Can you work these out from the drawing? Everything is in mm from the part's minimum corner. A direction names the side the tool comes from. Give positions to 0.01 mm unless a question says otherwise; leave off trailing zeros. Loops run counter-clockwise (first coordinate to the right, second up) from the corner with the lowest first, then second, coordinate; pieces in that order, holes last. Notation, with made-up numbers: (53, 30) - (81, 30) arc R17 ccw to (81, 63) - close; hole circle Ø9 at (52.25, -9). An arc over 180 degrees is marked (long way). One line per item, written item: value. Start each with the question number.
Q1. I want a section at C-C (x = 11.5). Please give me the cut outline in (y, z).
Q2. For the marked faces 1 and 2, which set-ups out of +Z, -Z, +X, -X, +Y, -Y let a thin tool reach every point of the face, with its end or its side?
Q3. I'm going to push flat-ended pins straight in: P1, Ø4, axis at y = 5.5, z = 64, coming from the +X side; P2, Ø6, axis at x = 16.5, y = 10.5, coming from the +Z side. Where does each tip first touch, or does it pass through?
Q4. If I drill on line 1 (Y direction, x = 22.5, z = 4.25); line 2 (X direction, y = 15, z = 48), over which ranges is the centre line in solid material (lowest first)? Write a range as from..to.
Q5. I want a section at D-D (z = 21.5). Please give me the cut outline in (x, y), then the cut area to 3 significant figures.
Q6. I want a section at A-A (x = 22.5). Please give me the cut outline in (y, z).
Q7. I want a section at B-B (y = 12.5). Please give me the cut outline in (x, z).
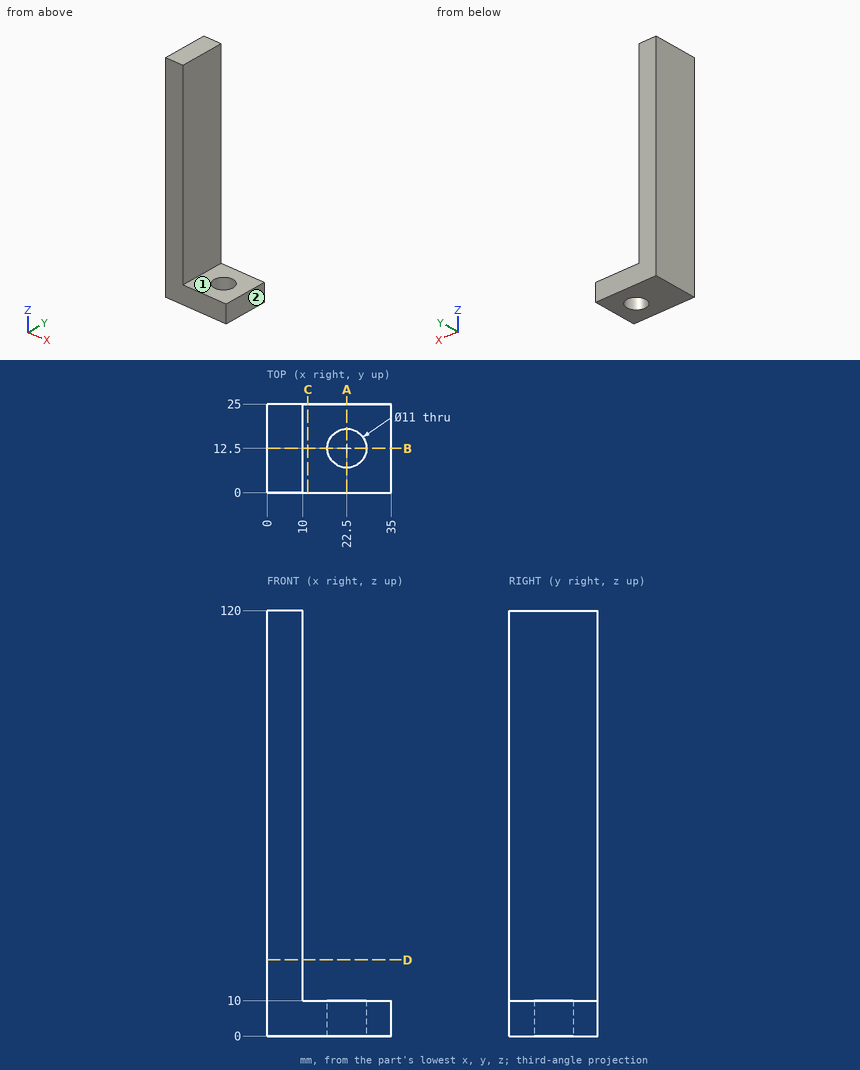
Worked answers:
1. outline: (0, 0) - (25, 0) - (25, 10) - (0, 10) - close
2. face 1: +Z, +X, +Y, -Y
2. face 2: +Z, -Z, +X, +Y, -Y
3. P1: stops at x = 10
3. P2: stops at z = 10
4. line 1: y = 0..7, 18..25
4. line 2: x = 0..10
5. outline: (0, 0) - (10, 0) - (10, 25) - (0, 25) - close
5. area: 250 mm²
6. outline: (0, 0) - (7, 0) - (7, 10) - (0, 10) - close; (18, 0) - (25, 0) - (25, 10) - (18, 10) - close
7. outline: (0, 0) - (17, 0) - (17, 10) - (10, 10) - (10, 120) - (0, 120) - close; (28, 0) - (35, 0) - (35, 10) - (28, 10) - close
